Check sheet for the modelled part. Datum: model origin and axes. Units: mm. Round coordinates to 2 decimals unless told otherwise and drop trailing zeros. Loops run counter-clockwise (first coordinate to the right, second up) from the corner with the lowest first, then second, coordinate; pieces in that order, holes last. Notation, with made-up numbers: (-30, -15) - (0, -15) arc R16 ccw to (0, -4) - close; hole circle Ø8 at (-32.75, 74.5). An arc over 180 degrees is marked (long way). Put each result on its own line as item: value. Start each with the question number.
Item 1: Section check B-B, the plane x = -91. Record the cut outline in (y, z), and give its area (3 significant figures).
Item 2: Material ranges on line 1 along X through (y, z) = (-32, 1.25); line 2 along X through (y, z) = (53.5, -0.75); line 3 along Z through (x, y) = (-136, 59), recorded low to high.
Item 3: Gauge pin test, flat ends, axial feed: pin 1 Ø2.5 at (y, z) = (-34.5, 1.5) entering from -X; pin 2 Ø1.5 at (x, y) = (83.5, -5.5) entering from -Z; pin 3 Ø3 at (y, z) = (48, -2.5) entering from +X. Record the tip position at first contact, or that the pin passes through.
Item 4: Section check A-A, the plane y = -26. Record the cut outline in (x, z), and give its area (4 significant figures).
Autodesk Inventor part; units mm, degrees
ref_plane "Work Plane1" through (0, 0, -5) normal (0, 0, 1) x (1, 0, 0)
ref_plane "YZ Plane" through (0, 0, 0) normal (1, 0, 0) x (0, 1, 0)
ref_plane "XZ Plane" through (0, 0, 0) normal (0, 1, 0) x (-1, 0, 0)
sketch "Sketch1" plane through (0, 0, 0) normal (0, 0, 1) x (1, 0, 0)
  line L0 (-177.5, 65) -> (177.5, 65)
  line L1 (177.5, 65) -> (177.5, -65)
  line L2 (177.5, -65) -> (-177.5, -65)
  line L3 (-177.5, -65) -> (-177.5, 65)
  line L4 (-177.5, 65) -> (177.5, -65) construction
  line L5 (177.5, 65) -> (-177.5, -65) construction
  point P0 (0, 0)
  dimension "d0" = 355
  dimension "d1" = 130
extrude "Extrusion1" add sketch "Sketch1" against normal blind 10
sketch "Sketch2" plane through (0, 0, 0) normal (0, 0, 1) x (1, 0, 0)
  line L0 (-162.5, 55) -> (-109.5, 55)
  line L1 (-104.5, 50) -> (-104.5, 9.1977)
  line L2 (-109.5, 4.1977) -> (-162.5, 4.1977)
  line L3 (-167.5, 9.1977) -> (-167.5, 50)
  line L4 (-177.5, 65) -> (177.5, 65)
  line L5 (-177.5, -65) -> (-177.5, 65)
  arc A0 (-162.5, 55) -> (-167.5, 50) centre (-162.5, 50) ccw
  arc A1 (-104.5, 50) -> (-109.5, 55) centre (-109.5, 50) ccw
  arc A2 (-109.5, 4.1977) -> (-104.5, 9.1977) centre (-109.5, 9.1977) ccw
  arc A3 (-167.5, 9.1977) -> (-162.5, 4.1977) centre (-162.5, 9.1977) ccw
  line L6 (-94.5, 55) -> (-41.5, 55)
  line L7 (-36.5, 50) -> (-36.5, 9.1977)
  line L8 (-41.5, 4.1977) -> (-94.5, 4.1977)
  line L9 (-99.5, 9.1977) -> (-99.5, 50)
  arc A4 (-94.5, 55) -> (-99.5, 50) centre (-94.5, 50) ccw
  arc A5 (-36.5, 50) -> (-41.5, 55) centre (-41.5, 50) ccw
  arc A6 (-41.5, 4.1977) -> (-36.5, 9.1977) centre (-41.5, 9.1977) ccw
  arc A7 (-99.5, 9.1977) -> (-94.5, 4.1977) centre (-94.5, 9.1977) ccw
  line L10 (-26.5, 55) -> (26.5, 55)
  line L11 (31.5, 50) -> (31.5, 9.1977)
  line L12 (26.5, 4.1977) -> (-26.5, 4.1977)
  line L13 (-31.5, 9.1977) -> (-31.5, 50)
  arc A8 (-26.5, 55) -> (-31.5, 50) centre (-26.5, 50) ccw
  arc A9 (31.5, 50) -> (26.5, 55) centre (26.5, 50) ccw
  arc A10 (26.5, 4.1977) -> (31.5, 9.1977) centre (26.5, 9.1977) ccw
  arc A11 (-31.5, 9.1977) -> (-26.5, 4.1977) centre (-26.5, 9.1977) ccw
  line L14 (41.5, 55) -> (94.5, 55)
  line L15 (99.5, 50) -> (99.5, 9.1977)
  line L16 (94.5, 4.1977) -> (41.5, 4.1977)
  line L17 (36.5, 9.1977) -> (36.5, 50)
  arc A12 (41.5, 55) -> (36.5, 50) centre (41.5, 50) ccw
  arc A13 (99.5, 50) -> (94.5, 55) centre (94.5, 50) ccw
  arc A14 (94.5, 4.1977) -> (99.5, 9.1977) centre (94.5, 9.1977) ccw
  arc A15 (36.5, 9.1977) -> (41.5, 4.1977) centre (41.5, 9.1977) ccw
  line L18 (109.5, 55) -> (162.5, 55)
  line L19 (167.5, 50) -> (167.5, 9.1977)
  line L20 (162.5, 4.1977) -> (109.5, 4.1977)
  line L21 (104.5, 9.1977) -> (104.5, 50)
  arc A16 (109.5, 55) -> (104.5, 50) centre (109.5, 50) ccw
  arc A17 (167.5, 50) -> (162.5, 55) centre (162.5, 50) ccw
  arc A18 (162.5, 4.1977) -> (167.5, 9.1977) centre (162.5, 9.1977) ccw
  arc A19 (104.5, 9.1977) -> (109.5, 4.1977) centre (109.5, 9.1977) ccw
  line L22 (-162.5, -5.802) -> (-109.5, -5.802)
  line L23 (-167.5, -51.6043) -> (-167.5, -10.802)
  line L24 (-109.5, -56.6043) -> (-162.5, -56.6043)
  line L25 (-104.5, -10.802) -> (-104.5, -51.6043)
  line L26 (-99.5, -51.6043) -> (-99.5, -10.802)
  line L27 (-94.5, -5.802) -> (-41.5, -5.802)
  line L28 (-36.5, -10.802) -> (-36.5, -51.6043)
  line L29 (-41.5, -56.6043) -> (-94.5, -56.6043)
  line L30 (-31.5, -51.6043) -> (-31.5, -10.802)
  line L31 (-26.5, -5.802) -> (26.5, -5.802)
  line L32 (31.5, -10.802) -> (31.5, -51.6043)
  line L33 (26.5, -56.6043) -> (-26.5, -56.6043)
  line L34 (41.5, -5.802) -> (94.5, -5.802)
  line L35 (36.5, -51.6043) -> (36.5, -10.802)
  line L36 (94.5, -56.6043) -> (41.5, -56.6043)
  line L37 (99.5, -10.802) -> (99.5, -51.6043)
  line L38 (104.5, -51.6043) -> (104.5, -10.802)
  line L39 (109.5, -5.802) -> (162.5, -5.802)
  line L40 (167.5, -10.802) -> (167.5, -51.6043)
  line L41 (162.5, -56.6043) -> (109.5, -56.6043)
  arc A20 (-162.5, -5.802) -> (-167.5, -10.802) centre (-162.5, -10.802) ccw
  arc A21 (-104.5, -10.802) -> (-109.5, -5.802) centre (-109.5, -10.802) ccw
  arc A22 (-167.5, -51.6043) -> (-162.5, -56.6043) centre (-162.5, -51.6043) ccw
  arc A23 (-109.5, -56.6043) -> (-104.5, -51.6043) centre (-109.5, -51.6043) ccw
  arc A24 (-99.5, -51.6043) -> (-94.5, -56.6043) centre (-94.5, -51.6043) ccw
  arc A25 (-94.5, -5.802) -> (-99.5, -10.802) centre (-94.5, -10.802) ccw
  arc A26 (-36.5, -10.802) -> (-41.5, -5.802) centre (-41.5, -10.802) ccw
  arc A27 (-26.5, -5.802) -> (-31.5, -10.802) centre (-26.5, -10.802) ccw
  arc A28 (-41.5, -56.6043) -> (-36.5, -51.6043) centre (-41.5, -51.6043) ccw
  arc A29 (-31.5, -51.6043) -> (-26.5, -56.6043) centre (-26.5, -51.6043) ccw
  arc A30 (31.5, -10.802) -> (26.5, -5.802) centre (26.5, -10.802) ccw
  arc A31 (26.5, -56.6043) -> (31.5, -51.6043) centre (26.5, -51.6043) ccw
  arc A32 (36.5, -51.6043) -> (41.5, -56.6043) centre (41.5, -51.6043) ccw
  arc A33 (41.5, -5.802) -> (36.5, -10.802) centre (41.5, -10.802) ccw
  arc A34 (99.5, -10.802) -> (94.5, -5.802) centre (94.5, -10.802) ccw
  arc A35 (94.5, -56.6043) -> (99.5, -51.6043) centre (94.5, -51.6043) ccw
  arc A36 (104.5, -51.6043) -> (109.5, -56.6043) centre (109.5, -51.6043) ccw
  arc A37 (109.5, -5.802) -> (104.5, -10.802) centre (109.5, -10.802) ccw
  arc A38 (167.5, -10.802) -> (162.5, -5.802) centre (162.5, -10.802) ccw
  arc A39 (162.5, -56.6043) -> (167.5, -51.6043) centre (162.5, -51.6043) ccw
  line L42 (171.5, 22) -> (183.5, 22)
  line L43 (183.5, 22) -> (183.5, -22)
  line L44 (183.5, -22) -> (171.5, -22)
  line L45 (171.5, -22) -> (171.5, 22)
  line L46 (177.5, 65) -> (177.5, -65)
  line L47 (171.5, 22) -> (183.5, -22) construction
  line L48 (183.5, 22) -> (171.5, -22) construction
  point P0 (0, 0)
  point P1 (-167.5, 55)
  point P2 (-104.5, 55)
  point P3 (-167.5, 4.1977)
  point P4 (-99.5, 55)
  point P5 (-36.5, 55)
  point P6 (-99.5, 4.1977)
  point P7 (-31.5, 55)
  point P8 (31.5, 55)
  point P9 (-31.5, 4.1977)
  point P10 (36.5, 55)
  point P11 (99.5, 55)
  point P12 (36.5, 4.1977)
  point P13 (104.5, 55)
  point P14 (167.5, 55)
  point P15 (104.5, 4.1977)
  point P16 (-167.5, -5.802)
  point P17 (-104.5, -5.802)
  point P18 (-167.5, -56.6043)
  point P19 (-99.5, -5.802)
  point P20 (-99.5, -56.6043)
  point P21 (-36.5, -5.802)
  point P22 (-31.5, -5.802)
  point P23 (-31.5, -56.6043)
  point P24 (31.5, -5.802)
  point P25 (36.5, -5.802)
  point P26 (99.5, -5.802)
  point P27 (36.5, -56.6043)
  point P28 (104.5, -5.802)
  point P29 (104.5, -56.6043)
  point P30 (167.5, -5.802)
  point P31 (177.5, 0)
  dimension "d4" = 10
  dimension "d5" = 10
  dimension "d7" = 50.8023
  dimension "d8" = 63
  dimension "d9" = 5
  dimension "d12" = 68
  dimension "d19" = 60.802
  dimension "d24" = 12
  dimension "d25" = 44
extrude "Extrusion2" add sketch "Sketch2" along normal blind 3 contours L0 A1 L1 A2 L2 A3 L3 A0 | L6 A5 L7 A6 L8 A7 L9 A4 | L10 A9 L11 A10 L12 A11 L13 A8 | L14 A13 L15 A14 L16 A15 L17 A12 | L18 A17 L19 A18 L20 A19 L21 A16 | L22 A21 L25 A23 L24 A22 L23 A20 | L26 A25 L27 A26 L28 A28 L29 A24 | L30 A27 L31 A30 L32 A31 L33 A29 | L34 A34 L37 A35 L36 A32 L35 A33 | L38 A37 L39 A38 L40 A39 L41 A36
ref_plane "Work Plane1" through (0, 0, -5) normal (0, 0, 1) x (1, 0, 0)
sketch "Sketch3" plane through (0, 0, -5) normal (0, 0, 1) x (1, 0, 0)
  line L0 (171.5, 22) -> (183.5, 22)
  line L1 (183.5, 22) -> (183.5, -22)
  line L2 (183.5, -22) -> (171.5, -22)
  line L3 (171.5, -22) -> (171.5, 22)
  line L4 (177.5, 65) -> (177.5, -65)
  line L5 (171.5, 22) -> (183.5, -22) construction
  line L6 (183.5, 22) -> (171.5, -22) construction
  point P0 (0, 0)
  point P1 (177.5, 0)
  dimension "d31" = 12
  dimension "d32" = 44
extrude "Extrusion3" add sketch "Sketch3" along normal mid plane 14
properties part number "Solar_panel"
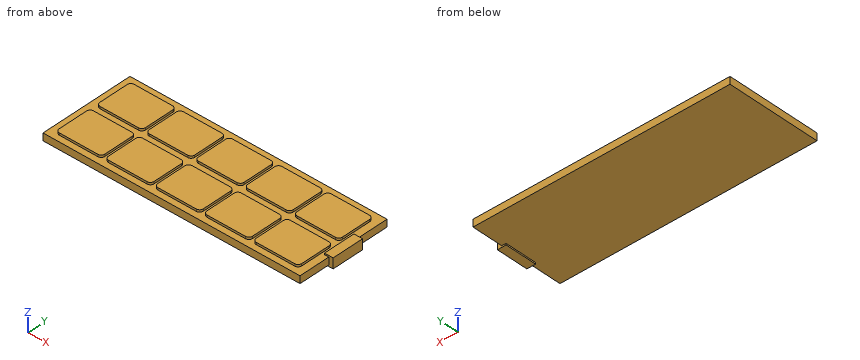
Check result:
1. outline: (-65, -10) - (65, -10) - (65, 0) - (55, 0) - (55, 3) - (4.2, 3) - (4.2, 0) - (-5.8, 0) - (-5.8, 3) - (-56.6, 3) - (-56.6, 0) - (-65, 0) - close
1. area: 1,600 mm²
2. line 1: -167.5 to -104.5, -99.5 to -36.5, -31.5 to 31.5, 36.5 to 99.5, 104.5 to 167.5
2. line 2: -177.5 to 177.5
2. line 3: -10 to 0
3. pin 1: x = -167.5
3. pin 2: z = -10
3. pin 3: x = 177.5
4. outline: (-177.5, -10) - (177.5, -10) - (177.5, 0) - (167.5, 0) - (167.5, 3) - (104.5, 3) - (104.5, 0) - (99.5, 0) - (99.5, 3) - (36.5, 3) - (36.5, 0) - (31.5, 0) - (31.5, 3) - (-31.5, 3) - (-31.5, 0) - (-36.5, 0) - (-36.5, 3) - (-99.5, 3) - (-99.5, 0) - (-104.5, 0) - (-104.5, 3) - (-167.5, 3) - (-167.5, 0) - (-177.5, 0) - close
4. area: 4,495 mm²
